Read the model definition and answer for the solid it produces. Units are mm, in the model's axes. A direction names the side the tool comes from. Coordinates: 2 decimals unless noted, no trailing zeros. Loops run counter-clockwise (first coordinate to the right, second up) from the corner with the lowest first, then second, coordinate; pieces in that order, holes last.
from build123d import *

# Parameters (mm, degrees)
ESBO_O3_R                  = 1.5
CORTE_EXTRUS_O1_DEPTH      = 1.8
CORTE_EXTRUS_O2_DEPTH      = 24.74931578
CORTE_EXTRUS_O2_DEPTH_BACK = 24.74931578
FILETE1_R                  = 0.2
ESBO_O12_R                 = 4.66979075
CORTE_EXTRUS_O3_DEPTH      = 4
ESBO_O15_R                 = 2.353382699
RESSALTO_EXTRUS_O2_DEPTH   = 1
FILETE2_R                  = 0.13
CORTE_EXTRUS_O4_DEPTH      = 20.400515457
CORTE_EXTRUS_O4_DEPTH_BACK = 20.400515457
ESBO_O16_R                 = 2.48
ESBO_O18_R                 = 2.48
RESSALTO_EXTRUS_O3_DEPTH   = 1.5
ESBO_O19_R                 = 0.75
RESSALTO_EXTRUS_O4_DEPTH   = 4
FILETE3_R                  = 0.5
ESBO_O20_R                 = 1.799226356
CORTE_EXTRUS_O5_DEPTH      = 10


with BuildPart() as part:
    # Esboço1 → Revolução1 (revolve)
    with BuildSketch(Plane.XY, mode=Mode.PRIVATE) as revolu_o1_sk:
        with BuildLine():
            Line((-3.37, 10.501320708), (-3.41, 10.501320708))
            Line((-3.41, 10.501320708), (-3.41, 8.101320708))
            Line((-3.41, 8.101320708), (-3.37, 8.101320708))
            Line((-3.37, 8.101320708), (-3.37, 4.101320708))
            Line((-3.37, 4.101320708), (-2.725, 2.329197773))
            Line((-2.725, 2.329197773), (-2.725, 0))
            Line((-2.725, 0), (0, 0))
            Line((0, 0), (0, 23.1))
            Line((0, 23.1), (-3.225, 23.1))
            ThreePointArc((-3.225, 23.1), (-3.578553391, 22.953553391), (-3.725, 22.6))
            Line((-3.725, 22.6), (-3.9, 22.6))
            Line((-3.9, 22.6), (-3.9, 18.6))
            Line((-3.9, 18.6), (-3.37, 18.6))
            Line((-3.37, 18.6), (-3.37, 15.8))
            Line((-3.37, 15.8), (-3.43, 15.8))
            Line((-3.43, 15.8), (-3.43, 13.4))
            Line((-3.43, 13.4), (-3.37, 13.4))
            Line((-3.37, 13.4), (-3.37, 10.501320708))
        make_face()
    revolve(revolu_o1_sk.sketch.rotate(Axis((0, 0, 0), (0, 1, 0)), 180), axis=Axis((0, 0, 0), (0, 1, 0)))

    # Esboço3 → Corte-extrusão1 (cut)
    with BuildSketch(Plane.XZ):
        Circle(ESBO_O3_R)
    extrude(amount=-CORTE_EXTRUS_O1_DEPTH, mode=Mode.SUBTRACT)

    # Esboço5 → Corte-extrusão2 (cut, two sides: drawn at the far end of the back side and taken through both)
    with BuildSketch(Plane(origin=(0, 0, 0), x_dir=(0, 0, -1), z_dir=(1, 0, 0)).offset(-CORTE_EXTRUS_O2_DEPTH_BACK)):
        Polygon((-0.589187623, 0), (0.589187623, 0), (0.4, 1.8), (-0.4, 1.8), align=None)
    extrude(amount=CORTE_EXTRUS_O2_DEPTH + CORTE_EXTRUS_O2_DEPTH_BACK, mode=Mode.SUBTRACT)

    # Esboço6 → Corte-Revolução1 (revolve, cut)
    with BuildSketch(Plane.XY, mode=Mode.PRIVATE) as corte_revolu_o1_sk:
        with BuildLine():
            Line((2.810516533, 23.1), (0, 23.1))
            Line((0, 23.1), (0, 22.6))
            Line((0, 22.6), (0, 3.9))
            ThreePointArc((0, 3.9), (0.790569415, 3.771708245), (1.5, 3.4))
            Line((1.5, 3.4), (1.75, 3.4))
            Line((1.75, 3.4), (1.75, 6.491111566))
            Line((1.75, 6.491111566), (2.45, 9.103547132))
            Line((2.45, 9.103547132), (2.45, 9.822456454))
            Line((2.45, 9.822456454), (2.26, 10.9))
            Line((2.26, 10.9), (2.46, 10.9))
            Line((2.46, 10.9), (2.46, 12.094100045))
            Line((2.46, 12.094100045), (2.265, 13.2))
            Line((2.265, 13.2), (2.465, 13.2))
            Line((2.465, 13.2), (2.48, 16.765743636))
            Line((2.48, 16.765743636), (2.28, 17.9))
            Line((2.28, 17.9), (2.48, 17.9))
            Line((2.48, 17.9), (2.48, 22.6))
            ThreePointArc((2.48, 22.6), (2.575060985, 22.819089023), (2.8, 22.899332591))
            Line((2.8, 22.899332591), (2.810516533, 23.1))
        make_face()
    revolve(corte_revolu_o1_sk.sketch.rotate(Axis((0, 22.6, 0), (0, -1, 0)), 180), axis=Axis((0, 22.6, 0), (0, -1, 0)), mode=Mode.SUBTRACT)

    # Filete1
    filete1_edges = [part.edges().sort_by_distance(p)[0] for p in [
        (1.75, 3.4, 0),
    ]]
    fillet(filete1_edges, radius=FILETE1_R)

    # Esboço9 → Corte-Revolução2 (revolve, cut)
    with BuildSketch(Plane.XY, mode=Mode.PRIVATE) as corte_revolu_o2_sk:
        Polygon((-6.004910607, 22.6), (-3.9, 22.6), (-3.9, 18.6), (-3.37, 18.6), (-3.37, 15.8), (-3.41, 15.8), (-3.41, 13.4), (-3.37, 13.4), (-3.37, 8.491421612), (-3.33, 8.381522515), (-3.33, 3.991421612), (-2.725, 2.329197773), (-6.004910607, 2.329197773), align=None)
    revolve(corte_revolu_o2_sk.sketch.rotate(Axis((0, 0, 0), (0, 1, 0)), 270), axis=Axis((0, 0, 0), (0, 1, 0)), mode=Mode.SUBTRACT)

    # Esboço12 → Corte-extrusão3 (cut)
    with BuildSketch(Plane.XZ):
        Circle(ESBO_O12_R)
    extrude(amount=-CORTE_EXTRUS_O3_DEPTH, mode=Mode.SUBTRACT)

    # Esboço15 → Ressalto-extrusão2 (add)
    with BuildSketch(Plane(origin=(0, 4.5, 0), x_dir=(-1, 0, 0), z_dir=(0, -1, 0))):
        Circle(ESBO_O15_R)
    extrude(amount=-RESSALTO_EXTRUS_O2_DEPTH)

    # Filete2
    filete2_edges = [part.edges().sort_by_distance(p)[0] for p in [
        (1.75, 4, 0),
        (0, 4, 3.33),
        (1.75, 6.491111566, 0),
        (2.45, 9.103547132, 0),
    ]]
    fillet(filete2_edges, radius=FILETE2_R)

    # Esboço16 → Corte-extrusão4 (cut, two sides: drawn at the far end of the back side and taken through both)
    with BuildSketch(Plane.XZ.offset(-4.5).offset(-CORTE_EXTRUS_O4_DEPTH_BACK)):
        with Locations(Location((0, 0, 0), (0, 0, 180))):
            Circle(ESBO_O16_R)
    extrude(amount=CORTE_EXTRUS_O4_DEPTH + CORTE_EXTRUS_O4_DEPTH_BACK, mode=Mode.SUBTRACT)

    # Esboço18 → Ressalto-extrusão3 (add)
    with BuildSketch(Plane(origin=(0, 8, 0), x_dir=(-1, 0, 0), z_dir=(0, -1, 0))):
        Circle(ESBO_O18_R)
    extrude(amount=-RESSALTO_EXTRUS_O3_DEPTH)

    # Esboço19 → Ressalto-extrusão4 (add)
    with BuildSketch(Plane.XZ.offset(-8)):
        Circle(ESBO_O19_R)
    extrude(amount=RESSALTO_EXTRUS_O4_DEPTH)

    # Filete3
    filete3_edges = [part.edges().sort_by_distance(p)[0] for p in [
        (-0.75, 4, 0),
    ]]
    fillet(filete3_edges, radius=FILETE3_R)

    # Esboço20 → Corte-extrusão5 (cut)
    with BuildSketch(Plane(origin=(0, 9.5, 0), x_dir=(1, 0, 0), z_dir=(0, 1, 0))):
        with Locations(Location((0, 0, 0), (0, 0, 180))):
            Circle(ESBO_O20_R)
    extrude(amount=-CORTE_EXTRUS_O5_DEPTH, mode=Mode.SUBTRACT)


solid = part.part
Item 1: Determine the mould class of faces 1 (the face through (-3, 18.6, 2)), 2 (the face through (0.54, 16.14, 2.42)), 3 (the face through (3.33, 14.58, 0.74)) for opening direction Z: released by +Z, released by -Z, zero draft, split by the parting line, or undercut.
Numbers:
face 1: zero draft
face 2: undercut
face 3: split by the parting line
Item 2: A cutting plane is placed at B-B on y = 19.5. Determine the outline of the cut face in (x, z).
Numbers:
outline: circle Ø7.8 at (0, 0); hole circle Ø4.96 at (0, 0)
Item 3: Find the intervals of material crossed by line 1 along Z through (x, y) = (0, 8.8); line 2 along Z through (x, y) = (0, 18); line 3 along Y through (x, z) = (1.5, -1.25), in increasing order.
Numbers:
line 1: z = -3.37 to -1.8, 1.8 to 3.37
line 2: z = -3.37 to -2.48, 2.48 to 3.37
line 3: y = 8 to 9.5
Item 4: A cutting plane is placed at A-A on y = 13.75. Determine the outline of the cut face in (x, z).
Numbers:
outline: circle Ø6.82 at (0, 0); hole circle Ø4.96 at (0, 0)
Item 5: Which of the six approach directions +Z, -Z, +X, -X, +Y, -Y give full straight-line access (tool end or side, diameter ignored) to faces 4 (the face through (3.13, 10.91, -1.25)), 5 (the face through (3.214, 17.18, -1.012)), 6 (the face through (2, 4, -2)), 7 (the face through (-2, 9.5, -1))?
Numbers:
face 4: -Y
face 5: none
face 6: +Z, -Z, +X, -X, -Y
face 7: +Y
Item 6: Given pin 1 (1 mm diameter, centred on y = 12.5, z = 0.5, fed in from +X); pin 2 (2 mm diameter, centred on x = 2, y = 19.5, fed in from +Z); pin 3 (1.5 mm diameter, centred on x = 1, z = 1, fed in from -Y), each flat-ended and moving along its own axis, determine where each tip first touches the part or whether it passes through.
Numbers:
pin 1: stops at x = 3.37
pin 2: stops at z = 3.77
pin 3: stops at y = 8
